Design review of the part shown in the three views and the two pictorial views. Dimensions are in mm from the part's minimum x, y and z. Coordinates: 2 decimals unless noted, no trailing zeros. Loops run counter-clockwise (first coordinate to the right, second up) from the corner with the lowest first, then second, coordinate; pieces in that order, holes last. Notation, with made-up numbers: M 31,65 L 85,65 A14 cw 85,84 Z; hole C 80.5,8 d5. An arc over 180 degrees is marked long. Use one line per item in the form item = value.
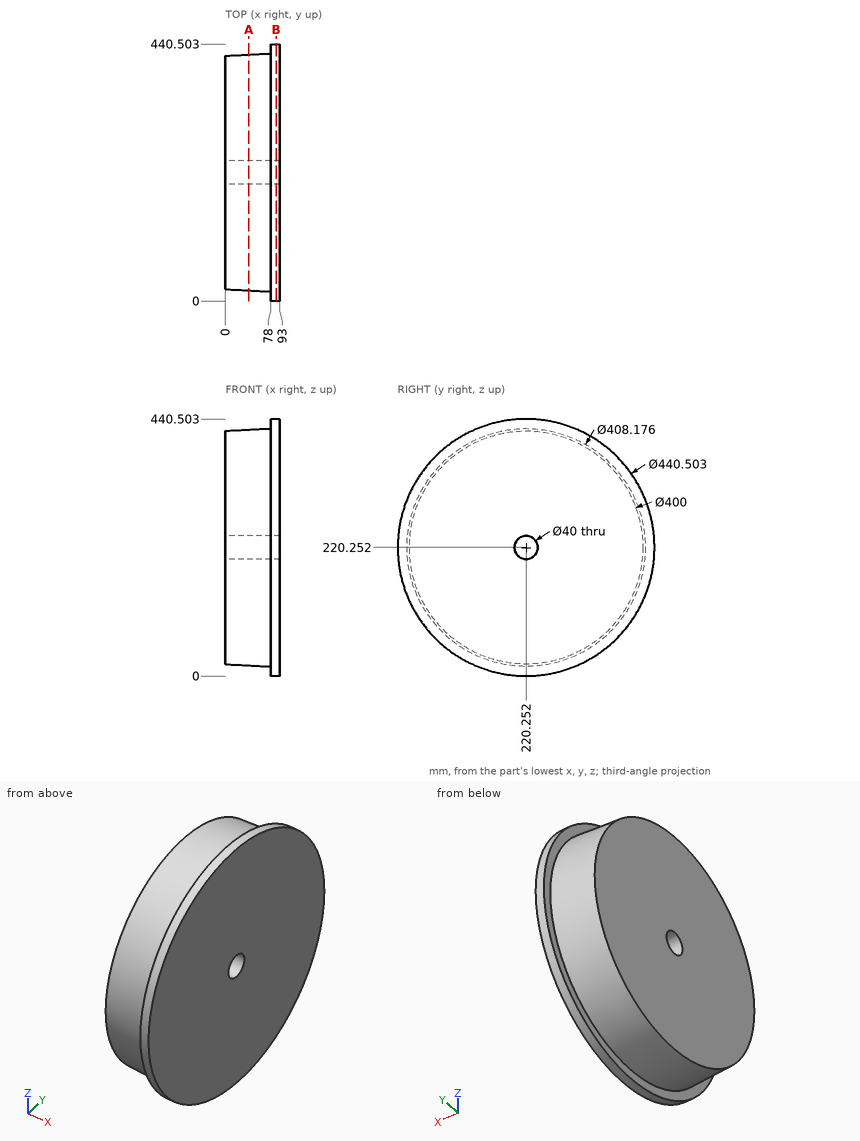
1. Wall thickness on line 1 along Y through (x, z) = (35.5, 204) (1 decimal); line 2 along X through (y, z) = (392, 352); line 3 along Z through (x, y) = (75, 213): over which ranges is each line inside the solid? List them lowest first. Write a range as from..to.
Response values:
line_1 = 19..208.6, 231.9..421.5
line_2 = 78..93
line_3 = 16.45..201.61, 238.89..424.05
2. Add section B-B (x = 87). State the section outline as (y, z) points, then the cut area to 3 significant figures.
Response values:
outline = C 220.25,220.25 d440.5; hole C 220.25,220.25 d40
area = 151,000 mm^2
3. Insertion check: P1, Ø3, axis at x = 38.5, y = 261, coming from the -Z side; P2, Ø1, axis at x = 37, z = 387.5, coming from the +Y side. Each pin has a flat end and moves straight along its axis. Give the tip position at first contact, or say it passes through.
Response values:
P1 = 22.07
P2 = 334.16
4. Add section A-A (x = 40.5). State the section outline as (y, z) points (1 decimal).
Response values:
outline = C 220.3,220.3 d404.2; hole C 220.3,220.3 d40
